from build123d import *

# Parameters (mm, degrees)
CROQUIS1_R              = 1
SALIENTE_EXTRUIR1_DEPTH = 4
CROQUIS3_R              = 1.25
CORTAR_EXTRUIR1_DEPTH   = 4
SALIENTE_EXTRUIR2_START = -4
CROQUIS4_R              = 3
SALIENTE_EXTRUIR2_DEPTH = 4
REDONDEO1_R             = 3
REDONDEO2_R             = 1.6
CROQUIS5_R              = 1.6
CORTAR_EXTRUIR2_DEPTH   = 4
CROQUIS6_R              = 1
CORTAR_EXTRUIR3_DEPTH   = 4


with BuildPart() as part:
    # Croquis1 → Saliente-Extruir1 (new body)
    with BuildSketch(Plane.XY):
        with BuildLine():
            Line((-15, -10.656453444), (-15, -40.656453444))
            Line((-15, -40.656453444), (15, -40.656453444))
            Line((15, -40.656453444), (15, -10.656453444))
            ThreePointArc((15, -10.656453444), (0, 18.4), (-15, -10.656453444))
        make_face()
        with Locations((-6.72, 10)):
            Circle(CROQUIS1_R, mode=Mode.SUBTRACT)
        with Locations((6.72, 10)):
            Circle(CROQUIS1_R, mode=Mode.SUBTRACT)
        with Locations((-6.72, 7.9)):
            Circle(CROQUIS1_R, mode=Mode.SUBTRACT)
        with Locations((6.72, 7.9)):
            Circle(CROQUIS1_R, mode=Mode.SUBTRACT)
        with Locations((-6.72, 5.8)):
            Circle(CROQUIS1_R, mode=Mode.SUBTRACT)
        with Locations((6.72, 5.8)):
            Circle(CROQUIS1_R, mode=Mode.SUBTRACT)
        with Locations((-6.72, 3.7)):
            Circle(CROQUIS1_R, mode=Mode.SUBTRACT)
        with Locations((6.72, 3.7)):
            Circle(CROQUIS1_R, mode=Mode.SUBTRACT)
        with Locations((-6.72, 1.6)):
            Circle(CROQUIS1_R, mode=Mode.SUBTRACT)
        with Locations((6.72, 1.6)):
            Circle(CROQUIS1_R, mode=Mode.SUBTRACT)
        with Locations((-6.72, -0.5)):
            Circle(CROQUIS1_R, mode=Mode.SUBTRACT)
        with Locations((6.72, -0.5)):
            Circle(CROQUIS1_R, mode=Mode.SUBTRACT)
        with Locations((-6.72, -2.6)):
            Circle(CROQUIS1_R, mode=Mode.SUBTRACT)
        with Locations((6.72, -2.6)):
            Circle(CROQUIS1_R, mode=Mode.SUBTRACT)
        with Locations((-6.72, -4.7)):
            Circle(CROQUIS1_R, mode=Mode.SUBTRACT)
        with Locations((6.72, -4.7)):
            Circle(CROQUIS1_R, mode=Mode.SUBTRACT)
        with Locations((-6.72, -6.8)):
            Circle(CROQUIS1_R, mode=Mode.SUBTRACT)
        with Locations((6.72, -6.8)):
            Circle(CROQUIS1_R, mode=Mode.SUBTRACT)
        with Locations((-6.72, -8.9)):
            Circle(CROQUIS1_R, mode=Mode.SUBTRACT)
        with Locations((6.72, -8.9)):
            Circle(CROQUIS1_R, mode=Mode.SUBTRACT)
        with Locations((-6.72, -11)):
            Circle(CROQUIS1_R, mode=Mode.SUBTRACT)
        with Locations((6.72, -11)):
            Circle(CROQUIS1_R, mode=Mode.SUBTRACT)
        with Locations((-6.72, -13.1)):
            Circle(CROQUIS1_R, mode=Mode.SUBTRACT)
        with Locations((6.72, -13.1)):
            Circle(CROQUIS1_R, mode=Mode.SUBTRACT)
        with BuildLine():
            Line((3, 0), (3, 10))
            ThreePointArc((3, 10), (0, 13), (-3, 10))
            Line((-3, 10), (-3, 0))
            Line((-3, 0), (-3, -12.5))
            ThreePointArc((-3, -12.5), (0, -15.5), (3, -12.5))
            Line((3, -12.5), (3, 0))
        make_face(mode=Mode.SUBTRACT)
    extrude(amount=SALIENTE_EXTRUIR1_DEPTH)

    # Croquis3 → Cortar-Extruir1 (cut)
    with BuildSketch(Plane.XZ.offset(40.656453444)):
        with Locations(Location((-10, 2, 0), (0, 0, 270))):
            Circle(CROQUIS3_R)
        with Locations(Location((10, 2, 0), (0, 0, 90))):
            Circle(CROQUIS3_R)
    extrude(amount=-CORTAR_EXTRUIR1_DEPTH, mode=Mode.SUBTRACT)

    # Croquis4 → Saliente-Extruir2 (add)
    with BuildSketch(Plane.XY.offset(4).offset(SALIENTE_EXTRUIR2_START)):
        with BuildLine():
            Line((5, 31.4), (-5, 31.4))
            Line((-5, 31.4), (-5, 17.707625476))
            ThreePointArc((-5, 17.707625476), (0, 18.4), (5, 17.707625476))
            Line((5, 17.707625476), (5, 31.4))
        make_face()
        with Locations((0, 26.4)):
            Circle(CROQUIS4_R, mode=Mode.SUBTRACT)
    extrude(amount=SALIENTE_EXTRUIR2_DEPTH)

    # Redondeo1
    redondeo1_edges = [part.edges().sort_by_distance(p)[0] for p in [
        (-5, 31.4, 2),
        (5, 31.4, 2),
    ]]
    fillet(redondeo1_edges, radius=REDONDEO1_R)

    # Redondeo2
    redondeo2_edges = [part.edges().sort_by_distance(p)[0] for p in [
        (-5, 17.707625476, 2),
        (5, 17.707625476, 2),
        (15, -10.656453444, 2),
        (-15, -10.656453444, 2),
    ]]
    fillet(redondeo2_edges, radius=REDONDEO2_R)

    # Croquis5 → Cortar-Extruir2 (cut)
    with BuildSketch(Plane.XY.offset(4)):
        with Locations((-10, -41.656453444)):
            Circle(CROQUIS5_R)
        with Locations((10, -41.656453444)):
            Circle(CROQUIS5_R)
    extrude(amount=-CORTAR_EXTRUIR2_DEPTH, mode=Mode.SUBTRACT)

    # Croquis6 → Cortar-Extruir3 (cut)
    with BuildSketch(Plane.XY.offset(4)):
        with Locations((0, -31.156453444)):
            Circle(CROQUIS6_R)
    extrude(amount=-CORTAR_EXTRUIR3_DEPTH, mode=Mode.SUBTRACT)


solid = part.part
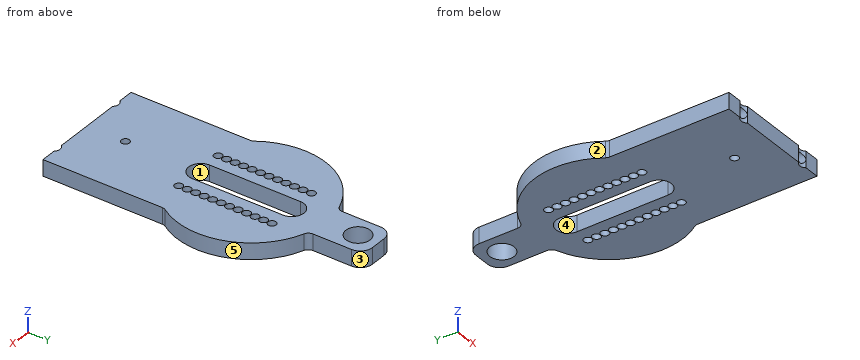
Verification items for the finished model (mm, model axes). Face numbers are marked on the shaded views. A direction names the side the tool comes from. Give positions to 0.01 mm unless a question says otherwise; leave off trailing zeros. Loops run counter-clockwise (first coordinate to the right, second up) from the corner with the lowest first, then second, coordinate; pieces in that order, holes last.
1) Thickness scan on line 1 along Y through (x, z) = (0, 1); line 2 along Y through (x, z) = (-2, 0.65); line 3 along X through (y, z) = (-4, 1.6). Record the ranges inside material, lowest first.
2) Depth check by flat-ended pin: pin 1 Ø1.6 at (x, y) = (6.72, 10) entering from +Z; pin 2 Ø2.5 at (x, y) = (6.72, -8.9) entering from +Z; pin 3 Ø2 at (y, z) = (-20, 2.5) entering from +X. Enter the tip coordinate at first touch or a pass-through.
3) Draft check along Y on the marked faces 3, 4 and 5. Enter one of: pulls with the +Y half, pulls with the -Y half, needs draft (parallel to the pull), parting line crosses it, or undercut.
4) Sectioned sample at A-A, the plane y = 26.4. Enter the section's corners in (x, z), then the cut area to 3 significant figures.
5) Sectioned sample at C-C, the plane x = 10. Enter the section's corners in (y, z), then the cut area to 3 significant figures.
6) Sectioned sample at D-D, the plane y = -6.8. Enter the section's corners in (x, z).
7) Sectioned sample at B-B, the plane y = 7.9. Enter the section's corners in (x, z).
8) Set-up check for the marked faces 1 and 2: record each of +Z, -Z, +X, -X, +Y, -Y from which the full face is reachable in a straight line by a thin tool's end or side.
Answers:
1. line 1: y = -40.66 to -32.16, -30.16 to -15.5, 13 to 23.4, 29.4 to 31.4
1. line 2: y = -40.66 to -14.74, 12.24 to 24.16, 28.64 to 31.4
1. line 3: x = -17.96 to -7.43, -6.01 to -3, 3 to 6.01, 7.43 to 17.96
2. pin 1: passes through
2. pin 2: stops at z = 4
2. pin 3: stops at x = 15
3. face 3: pulls with the +Y half
3. face 4: undercut
3. face 5: parting line crosses it
4. outline: (-5, 0) - (-3, 0) - (-3, 4) - (-5, 4) - close; (3, 0) - (5, 0) - (5, 4) - (3, 4) - close
4. area: 16.0 mm2
5. outline: (-40.06, 0) - (15.45, 0) - (15.45, 4) - (-40.06, 4) - (-40.06, 3.25) - (-36.66, 3.25) - (-36.66, 0.75) - (-40.06, 0.75) - close
5. area: 214 mm2
6. outline: (-17.1, 0) - (-7.72, 0) - (-7.72, 4) - (-17.1, 4) - close; (-5.72, 0) - (-3, 0) - (-3, 4) - (-5.72, 4) - close; (3, 0) - (5.72, 0) - (5.72, 4) - (3, 4) - close; (7.72, 0) - (17.1, 0) - (17.1, 4) - (7.72, 4) - close
7. outline: (-16.62, 0) - (-7.72, 0) - (-7.72, 4) - (-16.62, 4) - close; (-5.72, 0) - (-3, 0) - (-3, 4) - (-5.72, 4) - close; (3, 0) - (5.72, 0) - (5.72, 4) - (3, 4) - close; (7.72, 0) - (16.62, 0) - (16.62, 4) - (7.72, 4) - close
8. face 1: +Z, -Z
8. face 2: +Z, -Z, -X
